Could you check a few things on this model? Use its own coordinates, in mm. A direction names the side the tool comes from. Give positions to 0.01 mm unless a question says otherwise; leave off trailing zeros. Order: outer loops, then holes, each group sorted by start corner. A loop starts at its lowest first (then second) coordinate and runs counter-clockwise, first axis right, second up. Notation, with made-up numbers: (27, -17) - (39, -17) arc R4 ccw to (39, -11) - close; hole circle Ø2 at (-24.75, 22.25). An arc over 180 degrees is marked (long way). Put each result on its own line as item: value.
from build123d import *

# Parameters (mm, degrees)
F0_W     = 6.15
F0_H     = 6.15
F1_DEPTH = 3
F2_R     = 0.5
F3_R     = 1.65
F4_DEPTH = 1.4
F5_R     = 0.1


with BuildPart() as f1:
    # F0 (on Top) → F1 (new body)
    with BuildSketch(Plane.XY):
        with Locations((3.075, -3.075)):
            Rectangle(F0_W, F0_H)
    extrude(amount=F1_DEPTH)

    # F2
    f2_edges = [f1.edges().sort_by_distance(p)[0] for p in [
        (0, 0, 1.5),
        (6.15, 0, 1.5),
        (0, -6.15, 1.5),
        (6.15, -6.15, 1.5),
    ]]
    fillet(f2_edges, radius=F2_R)

    # F3 (on face) → F4 (join)
    with BuildSketch(Plane(origin=(0, 0, 0), x_dir=(1, 0, 0), z_dir=(0, 0, -1))):
        with Locations((3.075, 3.075)):
            Circle(F3_R)
    extrude(amount=F4_DEPTH)

    # F5
    f5_edges = [f1.edges().sort_by_distance(p)[0] for p in [
        (1.425, -3.075, -1.4),
    ]]
    fillet(f5_edges, radius=F5_R)


solid = f1.part
1) Suppose I cut it at C-C, the plane z = -0.8. List the corners of the cut face in (x, y) for me (3 decimals), and give its area (3 significant figures).
Filled in:
outline: circle Ø3.3 at (3.075, -3.075)
area: 8.55 mm^2
2) Suppose I cut it at B-B, the plane y = -5. List the corners of the cut face in (x, z) for me, and give its area (4 significant figures).
Filled in:
outline: (0, 0) - (6.15, 0) - (6.15, 3) - (0, 3) - close
area: 18.45 mm^2
3) Suppose I cut it at A-A, the plane x = 1. List the corners of the cut face in (y, z) for me.
Filled in:
outline: (-6.15, 0) - (0, 0) - (0, 3) - (-6.15, 3) - close
4) Which directions (+Z, -Z, +X, -X, +Y, -Y) give clear straight access to the entire face, cutting with the end or side of a thin tool? Please do faces 1 (the flat face through (6.15, -3, 1)), 2 (the flat face through (4.4, -1.7, 0)).
Filled in:
face 1: +Z, -Z, +X, +Y, -Y
face 2: -Z
5) If I drill on line 1 (Z direction, x = 4.75, y = -1.5); line 2 (X direction, y = -0.25, z = 2.65); line 3 (X direction, y = -4.25, z = -1.05), over which ranges is the centre line in solid material (lowest first)? Write a range as [from, to].
Filled in:
line 1: z = [0, 3]
line 2: x = [0.07, 6.08]
line 3: x = [1.92, 4.23]
